Can you work these out from the model? Positions are in its coordinate system, mm. Round coordinates to 2 decimals unless told otherwise and drop trailing zeros. Loops run counter-clockwise (first coordinate to the right, second up) from the corner with the lowest first, then second, coordinate; pieces in that order, holes last. Notation, with made-up numbers: M 8,36.5 L 36,36.5 A26 ccw 36,65.5 Z; hole C 57,13 d4. An arc over 180 degrees is marked long. Return JSON: item names as keys, results as strings.
```python
from build123d import *

# Parameters (mm, degrees)
SKETCH1_W                                           = 45.5
SKETCH1_H                                           = 29.5
BOSS_EXTRUDE1_DEPTH                                 = 5.5
CUT_EXTRUDE1_REACH                                  = 38.062
SKETCH2_R                                           = 13
CSK_FOR_M2_COUNTERSUNK_FLAT_HEAD_SCREW1_D           = 2.4
CSK_FOR_M2_COUNTERSUNK_FLAT_HEAD_SCREW1_CSINK_D     = 5.4
CSK_FOR_M2_COUNTERSUNK_FLAT_HEAD_SCREW1_CSINK_ANGLE = 90
M2_TAPPED_HOLE1_D                                   = 1.6


with BuildPart() as part:
    # Sketch1 → Boss-Extrude1 (new body)
    with BuildSketch(Plane(origin=(0, 0, 0), x_dir=(1, 0, 0), z_dir=(0, 1, 0))):
        Rectangle(SKETCH1_W, SKETCH1_H)
    extrude(amount=BOSS_EXTRUDE1_DEPTH)

    # Sketch2 → Cut-Extrude1 (cut, up to next)
    with BuildSketch(Plane(origin=(-14.125, 14.125, 0), x_dir=(0, 0, 1), z_dir=(-0.707106781, 0.707106781, 0)), mode=Mode.PRIVATE) as cut_extrude1_sk1:
        with Locations((0, 1.413320728)):
            Circle(SKETCH2_R)
    cut_extrude1_tool1 = extrude(cut_extrude1_sk1.sketch, amount=-CUT_EXTRUDE1_REACH, mode=Mode.PRIVATE) & part.part
    add(cut_extrude1_tool1.solids().sort_by_distance((-13.125631, 15.124369, 0))[0], mode=Mode.SUBTRACT)

    # CSK for M2 Countersunk Flat Head Screw1 (through all)
    with Locations(Plane(origin=(0, 5.5, 0), x_dir=(1, 0, 0), z_dir=(0, 1, 0))):
        with Locations((-19.75, 11.75), (19.25, 11.75), (-19.75, -11.75), (19.25, -11.75)):
            CounterSinkHole(CSK_FOR_M2_COUNTERSUNK_FLAT_HEAD_SCREW1_D / 2, CSK_FOR_M2_COUNTERSUNK_FLAT_HEAD_SCREW1_CSINK_D / 2, counter_sink_angle=CSK_FOR_M2_COUNTERSUNK_FLAT_HEAD_SCREW1_CSINK_ANGLE)

    # M2 Tapped Hole1 (through all)
    with Locations(Plane(origin=(0, 5.5, 0), x_dir=(1, 0, 0), z_dir=(0, 1, 0))):
        with Locations((20.25, 7), (20.25, -7)):
            Hole(M2_TAPPED_HOLE1_D / 2)


solid = part.part
```
Q1. I'm going to push flat-ended pins straight in: pin 1 Ø10 at (x, z) = (-15.5, 0) entering from +Y; pin 2 Ø3 at (x, z) = (-19.75, -11.75) entering from +Y. Where does each tip first touch, or does it pass through?
Results:
{"pin 1": "stops at y = 4.11", "pin 2": "stops at y = 4.3"}
Q2. Suppose I cut it at A-A, the plane z = 7. Please give me the cut outline in (x, y).
Results:
{"outline": "M -22.75,0 L -13.49,0 L -18.99,5.5 L -22.75,5.5 Z; M 11.99,5.5 L 17.49,0 L 19.45,0 L 19.45,5.5 Z; M 21.05,0 L 22.75,0 L 22.75,5.5 L 21.05,5.5 Z"}
Q3. Suppose I cut it at D-D, the plane x = -19.75. State how many separate pieces and enclosed holes the cut face has, plus the area to 3 significant figures.
Results:
{"separate pieces": "3", "enclosed holes": "0", "area": "114 mm2"}
Q4. Thinking about a two-plate mould opening in X: for faces 1 (the flat face through (22.75, 3, 0)), 2 (the flat face through (0, 3, -14.75)), 3 (the cylindrical face through (1.351, 5.149, -12.604)), which applies, pulls with the +X half, pulls with the -X half, needs draft (parallel to the pull), parting line crosses it, or undercut?
Results:
{"face 1": "pulls with the +X half", "face 2": "needs draft", "face 3": "undercut"}
Q5. Suppose I cut it at B-B, the plane z = -5.25. Please give me the cut outline in (x, y).
Results:
{"outline": "M -22.75,0 L -14.82,0 L -20.32,5.5 L -22.75,5.5 Z; M 13.32,5.5 L 18.82,0 L 22.75,0 L 22.75,5.5 Z"}
Q6. Suppose I cut it at C-C, the plane z = 11.75. Please give me the cut outline in (x, y).
Results:
{"outline": "M -22.75,0 L -20.95,0 L -20.95,4 L -22.45,5.5 L -22.75,5.5 Z; M -18.55,0 L -5.87,0 L -11.37,5.5 L -17.05,5.5 L -18.55,4 Z; M 4.36,5.5 L 9.86,0 L 18.05,0 L 18.05,4 L 16.55,5.5 Z; M 20.45,0 L 22.75,0 L 22.75,5.5 L 21.95,5.5 L 20.45,4 Z"}
Q7. If I drill on line 1 along Z through (x, y) = (19.25, 3.2); line 2 along Z through (x, y) = (20, 2.35); line 3 along X through (y, z) = (2.85, -7), over which ranges is the centre line in solid material (lowest first)?
Results:
{"line 1": "z = -14.75 to -12.95, -10.55 to 10.55, 12.95 to 14.75", "line 2": "z = -14.75 to -12.69, -10.81 to -7.76, -6.24 to 6.24, 7.76 to 10.81, 12.69 to 14.75", "line 3": "x = -22.75 to -16.34, 14.64 to 19.45, 21.05 to 22.75"}
